```python
from build123d import *

# Parameters (mm, degrees)
F0_W     = 25.4
F0_H     = 25.4
F1_DEPTH = 2
F2_R     = 1.27
F3_ANGLE = 180
F4_R     = 3.175


with BuildPart() as f1:
    # F0 (on Top) → F1 (new body)
    with BuildSketch(Plane.XY):
        Rectangle(F0_W, F0_H)
    extrude(amount=F1_DEPTH)

    # F2 (on face) → F3 (revolve)
    with BuildSketch(Plane.XY.offset(2)):
        with Locations((3.81, 0)):
            Circle(F2_R)
    revolve(axis=Axis((0, 0, 2), (0, -1, 0)), revolution_arc=F3_ANGLE)

    # F4
    f4_edges = [f1.edges().sort_by_distance(p)[0] for p in [
        (12.7, -12.7, 1),
        (-12.7, -12.7, 1),
        (-12.7, 12.7, 1),
        (12.7, 12.7, 1),
    ]]
    fillet(f4_edges, radius=F4_R)


solid = f1.part
```
The listing builds one solid part. Answer for the finished solid, in the listing's coordinates (mm). Coordinates: 2 decimals unless noted, no trailing zeros. Loops run counter-clockwise (first coordinate to the right, second up) from the corner with the lowest first, then second, coordinate; pieces in that order, holes last. Notation, with made-up numbers: (73.5, -8.5) - (78.5, -8.5) arc R24 cw to (78.5, 14.5) - close; hole circle Ø10 at (23.25, 44.5). An arc over 180 degrees is marked (long way). Use a Markdown table: item, result. Add a question column.
1) Given pin 1 (4 mm diameter, centred on x = 1.5, z = 6.5, fed in from -Y); pin 2 (12 mm diameter, centred on x = -3, y = 6, fed in from +Z); pin 3 (4 mm diameter, centred on x = 9, y = -0.5, fed in from +Z), each flat-ended and moving along its own axis, determine where each tip first touches the part or whether it passes through.
2) Find the intervals of material crossed by line 1 (Z direction, x = -10.25, y = 8); line 2 (Z direction, x = -0.25, y = -0.25); line 3 (X direction, y = 11, z = 1), in increasing order.
3) The part is cut by section C-C, the plane y = -4.5. Give the vertices of the cut face in (x, z), and give its area (3 significant figures).
4) The part is cut by section B-B, the plane y = 0.5. Give the vertices of the cut face in (x, z).
5) The part is cut by section A-A, the plane x = 0. Give the vertices of the cut face in (y, z), and give its area (3 significant figures).
Here are the results:
| question | item | result |
|---|---|---|
| 1 | pin 1 | stops at y = -1.27 |
| 1 | pin 2 | stops at z = 6.95 |
| 1 | pin 3 | stops at z = 2 |
| 2 | line 1 | z = 0 to 2 |
| 2 | line 2 | z = 0 to 2, 4.55 to 7.05 |
| 2 | line 3 | x = -12.34 to 12.34 |
| 3 | outline | (-12.7, 0) - (12.7, 0) - (12.7, 2) - (-12.7, 2) - close |
| 3 | area | 50.8 mm^2 |
| 4 | outline | (-12.7, 0) - (12.7, 0) - (12.7, 2) - (4.98, 2) arc R4.98 ccw to (-4.98, 2) - (-12.7, 2) - close; hole (-2.64, 2) - (2.64, 2) arc R2.64 ccw to start |
| 5 | outline | (-12.7, 0) - (12.7, 0) - (12.7, 2) - (-12.7, 2) - close; circle Ø2.54 at (0, 5.81) |
| 5 | area | 55.9 mm^2 |
